Geometry: final body of the model. Coordinates: model frame, mm. A direction names the side the tool comes from. Give positions to 0.01 mm unless a question says otherwise; leave off trailing zeros. Write each loop counter-clockwise with the first axis right and the second up, starting at its lowest first coordinate (ties: lowest second). Pieces come first, ordered by that corner, then holes. Notation, with made-up numbers: M 81.5,75.25 L 136.5,75.25 A14 ccw 136.5,88.25 Z; hole C -34,-38.5 d5. An arc over 180 degrees is marked long. Use one line per item in the form item = value. Start each with the question number.
Item 1: Material intervals for line 1 along Y through (x, z) = (-68, 3); line 2 along X through (y, z) = (60, 6); line 3 along X through (y, z) = (53.5, 2.5), sorted ascending. Write a range as from..to.
Item 2: Pull-direction query (Y, two-part tool) for faces 1 (the flat face through (203, 111.473, 3)), 2 (the flat face through (15, 63, 3)), 3 (the flat face through (206.35, 102, 3)); classes: released by +Y, released by -Y, zero draft, split by the parting line, or undercut.
Item 3: Section query B-B on y = 128.5. Return loops of the section in (x, z).
Item 4: Access query for faces 4 (the flat face through (200, 3, 3)), 5 (the flat face through (125, 63, 3)), 6 (the flat face through (-153, 41.473, 3)), 7 (the flat face through (-153, 111.473, 3)). Directions: +Z, -Z, +X, -X, +Y, -Y. A direction counts if a zero-diameter tool reaches every point of the face in a straight line with its end or side. Return the directions, or none.
Item 5: Contact query for flat-ended pins moving along their axis: P1, Ø3, axis at y = 3.5, z = 1.5, coming from the -X side; P2, Ø1.9, axis at y = 141, z = 3, coming from the +X side; P3, Ø1.9, axis at x = 203, z = 2, coming from the +Y side. Output: stop coordinate, or through.
Item 6: Section query A-A on z = 2.75. Give the number of separate pieces and of enclosed holes in the cut face, then the cut area to 3 significant figures.
from build123d import *

# Parameters (mm, degrees)
CROQUIS1_W              = 350
CROQUIS1_H              = 201.8383275
SALIENTE_EXTRUIR1_DEPTH = 6.35
CROQUIS2_W              = 6.35
CROQUIS2_H              = 20
SALIENTE_EXTRUIR2_DEPTH = 6.35
CROQUIS3_W              = 20
CROQUIS3_H              = 6.35
CORTAR_EXTRUIR1_DEPTH   = 6.35
CROQUIS4_W              = 350
CROQUIS4_H              = 15
SALIENTE_EXTRUIR3_DEPTH = 6.35


with BuildPart() as part:
    # Croquis1 → Saliente-Extruir1 (new body)
    with BuildSketch(Plane.XY):
        with Locations((25, 100.551894806)):
            Rectangle(CROQUIS1_W, CROQUIS1_H)
    extrude(amount=SALIENTE_EXTRUIR1_DEPTH)

    # Croquis2 → Saliente-Extruir2 (add)
    with BuildSketch(Plane.ZY.offset(150)):
        with Locations((3.175, 31.472731056)):
            Rectangle(CROQUIS2_W, CROQUIS2_H)
        with Locations((3.175, 101.472731056)):
            Rectangle(CROQUIS2_W, CROQUIS2_H)
    saliente_extruir2 = extrude(amount=SALIENTE_EXTRUIR2_DEPTH)

    # Simetría1: Saliente-Extruir2 across plane
    add(saliente_extruir2.mirror(Plane(origin=(25, 0, 0), x_dir=(0, 0, 1), z_dir=(1, 0, 0))))

    # Croquis3 → Cortar-Extruir1 (cut)
    with BuildSketch(Plane(origin=(0, 0, 0), x_dir=(-1, 0, 0), z_dir=(0, 0, -1))):
        with Locations((-25, 2.807731056)):
            Rectangle(CROQUIS3_W, CROQUIS3_H)
        with Locations((65, 2.807731056)):
            Rectangle(CROQUIS3_W, CROQUIS3_H)
        with Locations((-115, 2.807731056)):
            Rectangle(CROQUIS3_W, CROQUIS3_H)
        with Locations((-25, 62.807731056)):
            Rectangle(CROQUIS3_W, CROQUIS3_H)
        with Locations((65, 62.807731056)):
            Rectangle(CROQUIS3_W, CROQUIS3_H)
        with Locations((-115, 62.807731056)):
            Rectangle(CROQUIS3_W, CROQUIS3_H)
    extrude(amount=-CORTAR_EXTRUIR1_DEPTH, mode=Mode.SUBTRACT)

    # Croquis4 → Saliente-Extruir3 (add)
    with BuildSketch(Plane.XY.offset(6.35)):
        with Locations((25, -7.867268944)):
            Rectangle(CROQUIS4_W, CROQUIS4_H)
    extrude(amount=-SALIENTE_EXTRUIR3_DEPTH)


solid = part.part
Answer sheet:
q1.line_1 = -15.37..-0.37, 5.98..59.63, 65.98..201.47
q1.line_2 = -150..-75, -55..15, 35..105, 125..200
q1.line_3 = -150..200
q2.face_1 = released by +Y
q2.face_2 = undercut
q2.face_3 = zero draft
q3.outline = M -150,0 L 200,0 L 200,6.35 L -150,6.35 Z
q4.face_4 = +Z, -Z, +X, -Y
q4.face_5 = +Z, -Z
q4.face_6 = +Z, -Z, -X
q4.face_7 = +Z, -Z, -X, +Y
q5.P1 = -150
q5.P2 = 200
q5.P3 = 111.47
q6.separate_pieces = 1
q6.enclosed_holes = 6
q6.area = 75,600 mm2
